The listing builds one solid part. Answer for the finished solid, in the listing's coordinates (mm). Round coordinates to 2 decimals unless told otherwise and drop trailing zeros. One line per item, written item: value. Start each with the question number.
(1) Section A-A (z = -44) is taken. State how many separate pieces and enclosed holes the cut face has, plus the area to 3 significant figures.
(2) Consider probe 1 along Y at (x, z) = (7.75, -354); probe 2 along Y at (x, z) = (-5, -528); probe 3 along Y at (x, z) = (0, -347.5). Determine where each line is inside the solid, lowest interval first.
(3) Given P1, Ø0.7, axis at y = 11.5, z = -356, coming from the -X side; P2, Ø0.6, axis at x = 9.5, z = -408.5, coming from the -Y side; P3, Ø0.7, axis at y = -12, z = -261, coming from the +X side, each flat-ended and moving along its own axis, determine where each tip first touches the part or whether it passes through.
```python
from build123d import *

# Parameters (mm, degrees)
BOSS_EXTRUDE1_DEPTH = 550
SKETCH2_W           = 550
SKETCH2_H           = 2.1
SKETCH3_W           = 550
SKETCH3_H           = 2.1


with BuildPart() as part:
    # Sketch1 → Boss-Extrude1 (new body)
    with BuildSketch(Plane.XY):
        with BuildLine():
            Line((-10, -7), (-8, -7))
            Line((-8, -7), (-8, -4))
            Line((-8, -4), (-7.060660172, -4))
            Line((-7.060660172, -4), (-4, -7.060660172))
            Line((-4, -7.060660172), (-4, -9.480384758))
            Line((-4, -9.480384758), (-3.7, -10))
            Line((-3.7, -10), (-4, -10.519615242))
            Line((-4, -10.519615242), (-4, -12.939339828))
            Line((-4, -12.939339828), (-7.060660172, -16))
            Line((-7.060660172, -16), (-8, -16))
            Line((-8, -16), (-8, -13))
            Line((-8, -13), (-10, -13))
            Line((-10, -13), (-10, -19))
            ThreePointArc((-10, -19), (-9.707106781, -19.707106781), (-9, -20))
            Line((-9, -20), (-3, -20))
            Line((-3, -20), (-3, -18))
            Line((-3, -18), (-6, -18))
            Line((-6, -18), (-6, -17.060660172))
            Line((-6, -17.060660172), (-2.939339828, -14))
            Line((-2.939339828, -14), (-0.519615242, -14))
            Line((-0.519615242, -14), (0, -13.7))
            Line((0, -13.7), (0.519615242, -14))
            Line((0.519615242, -14), (2.939339828, -14))
            Line((2.939339828, -14), (6, -17.060660172))
            Line((6, -17.060660172), (6, -18))
            Line((6, -18), (3, -18))
            Line((3, -18), (3, -20))
            Line((3, -20), (9, -20))
            ThreePointArc((9, -20), (9.707106781, -19.707106781), (10, -19))
            Line((10, -19), (10, -13))
            Line((10, -13), (8, -13))
            Line((8, -13), (8, -16))
            Line((8, -16), (7.060660172, -16))
            Line((7.060660172, -16), (4, -12.939339828))
            Line((4, -12.939339828), (4, -10.519615242))
            Line((4, -10.519615242), (3.7, -10))
            Line((3.7, -10), (4, -9.480384758))
            Line((4, -9.480384758), (4, -7.060660172))
            Line((4, -7.060660172), (7.060660172, -4))
            Line((7.060660172, -4), (8, -4))
            Line((8, -4), (8, -7))
            Line((8, -7), (10, -7))
            Line((10, -7), (10, 7))
            Line((10, 7), (8, 7))
            Line((8, 7), (8, 4))
            Line((8, 4), (7.060660172, 4))
            Line((7.060660172, 4), (4, 7.060660172))
            Line((4, 7.060660172), (4, 9.480384758))
            Line((4, 9.480384758), (3.7, 10))
            Line((3.7, 10), (4, 10.519615242))
            Line((4, 10.519615242), (4, 12.939339828))
            Line((4, 12.939339828), (7.060660172, 16))
            Line((7.060660172, 16), (8, 16))
            Line((8, 16), (8, 13))
            Line((8, 13), (10, 13))
            Line((10, 13), (10, 19))
            ThreePointArc((10, 19), (9.707106781, 19.707106781), (9, 20))
            Line((9, 20), (3, 20))
            Line((3, 20), (3, 18))
            Line((3, 18), (6, 18))
            Line((6, 18), (6, 17.060660172))
            Line((6, 17.060660172), (2.939339828, 14))
            Line((2.939339828, 14), (0.519615242, 14))
            Line((0.519615242, 14), (0, 13.7))
            Line((0, 13.7), (-0.519615242, 14))
            Line((-0.519615242, 14), (-2.939339828, 14))
            Line((-2.939339828, 14), (-6, 17.060660172))
            Line((-6, 17.060660172), (-6, 18))
            Line((-6, 18), (-3, 18))
            Line((-3, 18), (-3, 20))
            Line((-3, 20), (-9, 20))
            ThreePointArc((-9, 20), (-9.707106781, 19.707106781), (-10, 19))
            Line((-10, 19), (-10, 13))
            Line((-10, 13), (-8, 13))
            Line((-8, 13), (-8, 16))
            Line((-8, 16), (-7.060660172, 16))
            Line((-7.060660172, 16), (-4, 12.939339828))
            Line((-4, 12.939339828), (-4, 10.519615242))
            Line((-4, 10.519615242), (-3.7, 10))
            Line((-3.7, 10), (-4, 9.480384758))
            Line((-4, 9.480384758), (-4, 7.060660172))
            Line((-4, 7.060660172), (-7.060660172, 4))
            Line((-7.060660172, 4), (-8, 4))
            Line((-8, 4), (-8, 7))
            Line((-8, 7), (-10, 7))
            Line((-10, 7), (-10, -7))
        make_face()
        with BuildLine():
            Line((-8, 1.7), (-8, -1.7))
            ThreePointArc((-8, -1.7), (-7.912132034, -1.912132034), (-7.7, -2))
            Line((-7.7, -2), (-7.063603897, -2))
            ThreePointArc((-7.063603897, -2), (-6.948798867, -2.02283614), (-6.851471863, -2.087867966))
            Line((-6.851471863, -2.087867966), (-2.939339828, -6))
            Line((-2.939339828, -6), (2.939339828, -6))
            Line((2.939339828, -6), (6.851471863, -2.087867966))
            ThreePointArc((6.851471863, -2.087867966), (6.948798867, -2.02283614), (7.063603897, -2))
            Line((7.063603897, -2), (7.7, -2))
            ThreePointArc((7.7, -2), (7.912132034, -1.912132034), (8, -1.7))
            Line((8, -1.7), (8, 1.7))
            ThreePointArc((8, 1.7), (7.912132034, 1.912132034), (7.7, 2))
            Line((7.7, 2), (7.063603897, 2))
            ThreePointArc((7.063603897, 2), (6.948798867, 2.02283614), (6.851471863, 2.087867966))
            Line((6.851471863, 2.087867966), (2.939339828, 6))
            Line((2.939339828, 6), (-2.939339828, 6))
            Line((-2.939339828, 6), (-6.851471863, 2.087867966))
            ThreePointArc((-6.851471863, 2.087867966), (-6.948798867, 2.02283614), (-7.063603897, 2))
            Line((-7.063603897, 2), (-7.7, 2))
            ThreePointArc((-7.7, 2), (-7.912132034, 1.912132034), (-8, 1.7))
        make_face(mode=Mode.SUBTRACT)
    extrude(amount=-BOSS_EXTRUDE1_DEPTH)

    # Sketch2 → Cut-Revolve1 (revolve, cut)
    with BuildSketch(Plane(origin=(0, 0, 0), x_dir=(0, 0, -1), z_dir=(1, 0, 0)), mode=Mode.PRIVATE) as cut_revolve1_sk:
        with Locations((275, 11.05)):
            Rectangle(SKETCH2_W, SKETCH2_H)
    revolve(cut_revolve1_sk.sketch.rotate(Axis((0, 10, -550), (0, 0, 1)), 270), axis=Axis((0, 10, -550), (0, 0, 1)), mode=Mode.SUBTRACT)

    # Sketch3 → Cut-Revolve2 (revolve, cut)
    with BuildSketch(Plane(origin=(0, 0, 0), x_dir=(0, 0, -1), z_dir=(1, 0, 0)), mode=Mode.PRIVATE) as cut_revolve2_sk:
        with Locations((275, -8.95)):
            Rectangle(SKETCH3_W, SKETCH3_H)
    revolve(cut_revolve2_sk.sketch.rotate(Axis((0, -10, -550), (0, 0, 1)), 270), axis=Axis((0, -10, -550), (0, 0, 1)), mode=Mode.SUBTRACT)


solid = part.part
```
Recorded:
1. separate pieces: 1
1. enclosed holes: 3
1. area: 324 mm2
2. probe 1: y = -20 to -16, -4 to -2, 2 to 4, 16 to 20
2. probe 2: y = -20 to -18, -16.06 to -13.94, -6.06 to -3.94, 3.94 to 6.06, 13.94 to 16.06, 18 to 20
2. probe 3: y = -13.7 to -12.1, -7.9 to -6, 6 to 7.9, 12.1 to 13.7
3. P1: stops at x = -4
3. P2: stops at y = -19.98
3. P3: stops at x = 4
